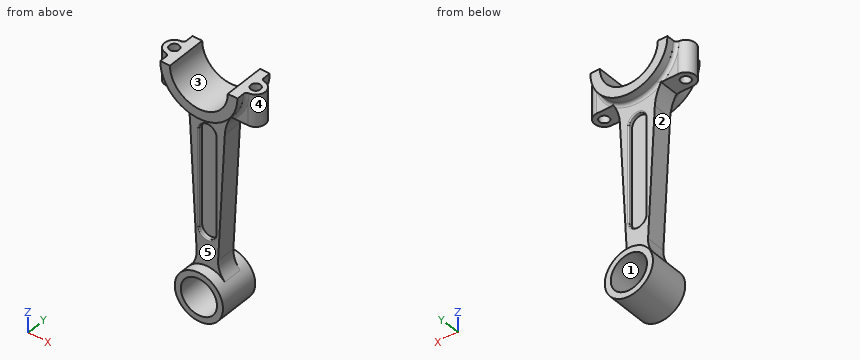
```python
from build123d import *

# Parameters (mm, degrees)
SKETCH1_R             = 22.5
SKETCH1_R_2           = 16.9
BOSS_EXTRUDE1_DEPTH   = 19
BOSS_EXTRUDE1_2_DEPTH = 19
BOSS_EXTRUDE2_DEPTH   = 9
BOSS_EXTRUDE3_DEPTH   = 5
FILLET2_R             = 1
BOSS_EXTRUDE4_DEPTH   = 9
FILLET3_R             = 3
SKETCH5_R             = 4.5
CUT_EXTRUDE1_DEPTH    = 38


with BuildPart() as part:
    # Sketch1 → Boss-Extrude1 (new, symmetric)
    with BuildSketch(Plane(origin=(0, 0, 0), x_dir=(1, 0, 0), z_dir=(0, 1, 0))):
        with Locations(Location((0, 201.2, 0), (0, 0, 270))):
            Circle(SKETCH1_R)
        with Locations(Location((0, 201.2, 0), (0, 0, 270))):
            Circle(SKETCH1_R_2, mode=Mode.SUBTRACT)
    extrude(amount=BOSS_EXTRUDE1_DEPTH, both=True)



with BuildPart() as body_2:
    # Sketch1 → Boss-Extrude1 2 (new, symmetric)
    with BuildSketch(Plane(origin=(0, 0, 0), x_dir=(1, 0, 0), z_dir=(0, 1, 0))):
        with BuildLine():
            Line((27, 0), (36, 0))
            ThreePointArc((36, 0), (0, 36), (-36, 0))
            Line((-36, 0), (-27, 0))
            ThreePointArc((-27, 0), (0, 27), (27, 0))
        make_face()
    extrude(amount=BOSS_EXTRUDE1_2_DEPTH, both=True)


with BuildPart() as part_1:
    add(part.part)

    add(body_2.part)  # Boss-Extrude2 merges body 2
    # Sketch1<3> → Boss-Extrude2 (add, symmetric)
    with BuildSketch(Plane(origin=(0, 0, 0), x_dir=(1, 0, 0), z_dir=(0, 1, 0))):
        with BuildLine():
            ThreePointArc((-16.279722223, 49.041287854), (-19.307974883, 35.735363352), (-26.63284908, 24.221712365))
            ThreePointArc((-26.63284908, 24.221712365), (0, 36), (26.63284908, 24.221712365))
            ThreePointArc((26.63284908, 24.221712365), (19.307974883, 35.735363352), (16.279722223, 49.041287854))
            Line((16.279722223, 49.041287854), (10, 168.865525948))
            ThreePointArc((10, 168.865525948), (11.381584619, 177.889356271), (16.234582266, 185.621542482))
            ThreePointArc((16.234582266, 185.621542482), (0, 178.7), (-16.234582266, 185.621542482))
            ThreePointArc((-16.234582266, 185.621542482), (-11.381584619, 177.889356271), (-10, 168.865525948))
            Line((-10, 168.865525948), (-16.279722223, 49.041287854))
        make_face()
        with BuildLine():
            ThreePointArc((8, 55.6), (0, 47.6), (-8, 55.6))
            Line((-8, 55.6), (-8, 145.6))
            ThreePointArc((-8, 145.6), (0, 153.6), (8, 145.6))
            Line((8, 145.6), (8, 55.6))
        make_face(mode=Mode.SUBTRACT)
    extrude(amount=BOSS_EXTRUDE2_DEPTH, both=True)

    # Sketch1<4> → Boss-Extrude3 (add, symmetric)
    with BuildSketch(Plane(origin=(0, 0, 0), x_dir=(1, 0, 0), z_dir=(0, 1, 0))):
        with BuildLine():
            Line((8, 55.6), (8, 145.6))
            ThreePointArc((8, 145.6), (0, 153.6), (-8, 145.6))
            Line((-8, 145.6), (-8, 55.6))
            ThreePointArc((-8, 55.6), (0, 47.6), (8, 55.6))
        make_face()
    extrude(amount=BOSS_EXTRUDE3_DEPTH, both=True)

    # Fillet2
    fillet2_edges = [part_1.edges().sort_by_distance(p)[0] for p in [
        (0, 9, -153.6),
        (8, 9, -100.6),
        (0, 9, -47.6),
        (-8, -9, -100.6),
        (-8, 9, -100.6),
        (0, -9, -153.6),
        (0, -9, -47.6),
        (8, -9, -100.6),
    ]]
    fillet(fillet2_edges, radius=FILLET2_R)

    # Sketch3 → Boss-Extrude4 (add, symmetric)
    with BuildSketch(Plane(origin=(0, 0, 0), x_dir=(1, 0, 0), z_dir=(0, 1, 0))):
        with BuildLine():
            Line((-19.899748742, 30), (-49, 30))
            Line((-49, 30), (-49, 0))
            Line((-49, 0), (-36, 0))
            ThreePointArc((-36, 0), (-31.720584442, 17.023645986), (-19.899748742, 30))
        make_face()
        with BuildLine():
            Line((49, 30), (49, 0))
            Line((49, 0), (36, 0))
            ThreePointArc((36, 0), (31.720584442, 17.023645986), (19.899748742, 30))
            Line((19.899748742, 30), (49, 30))
        make_face()
    extrude(amount=BOSS_EXTRUDE4_DEPTH, both=True)

    # Fillet3
    # the kernel refuses this fillet: 3 mm, written as the material it adds along each edge
    with BuildSketch(Plane(origin=(0, 9, 0), x_dir=(-1, 0, 0), z_dir=(0, 0, 1))) as fillet3_piece_1_section:
        with BuildLine():
            CenterArc((36 + FILLET3_R, -FILLET3_R), FILLET3_R, 90, 90)
            Line((36, -FILLET3_R), (36, 0))
            Line((36, 0), (36 + FILLET3_R, 0))
        make_face()
    fillet3_piece_1 = revolve(axis=Axis((0, 9, 0), (0, -1, 0)), revolution_arc=180, mode=Mode.PRIVATE)
    fillet3_piece_1 = split(fillet3_piece_1, bisect_by=Plane(origin=(-34.322989988, 9.698532199, -30), z_dir=(0, 0, 1)), keep=Keep.TOP, mode=Mode.PRIVATE)
    add(fillet3_piece_1)
    with BuildSketch(Plane(origin=(0, 9, 0), x_dir=(-1, 0, 0), z_dir=(0, 0, 1))) as fillet3_piece_2_section:
        with BuildLine():
            CenterArc((36 + FILLET3_R, -FILLET3_R), FILLET3_R, 90, 90)
            Line((36, -FILLET3_R), (36, 0))
            Line((36, 0), (36 + FILLET3_R, 0))
        make_face()
    fillet3_piece_2 = revolve(axis=Axis((0, 9, 0), (0, -1, 0)), revolution_arc=180, mode=Mode.PRIVATE)
    fillet3_piece_2 = fillet3_piece_2 - Plane(origin=(56.224903613, 10.5000003, -51.134726104), x_dir=(-0.7398013633284897, 0, 0.6728253434713263), z_dir=(0, 1, 0)) * Cylinder(40, 157, mode=Mode.PRIVATE)
    fillet3_piece_2 = fillet3_piece_2 - Plane(origin=(-56.224903613, 10.5000003, -51.134726104), x_dir=(0.9986295347545738, 0, 0.05233595624294564), z_dir=(0, 1, 0)) * Cylinder(40, 157, mode=Mode.PRIVATE)
    add(fillet3_piece_2)
    with BuildSketch(Plane(origin=(0, -9, 0), x_dir=(1, 0, 0), z_dir=(0, 0, 1))) as fillet3_piece_3_section:
        with BuildLine():
            CenterArc((36 + FILLET3_R, -FILLET3_R), FILLET3_R, 90, 90)
            Line((36, -FILLET3_R), (36, 0))
            Line((36, 0), (36 + FILLET3_R, 0))
        make_face()
    fillet3_piece_3 = revolve(axis=Axis((0, -9, 0), (0, 1, 0)), revolution_arc=180, mode=Mode.PRIVATE)
    fillet3_piece_3 = split(fillet3_piece_3, bisect_by=Plane(origin=(34.322988047, -9.698532268, -30), z_dir=(0, 0, 1)), keep=Keep.TOP, mode=Mode.PRIVATE)
    add(fillet3_piece_3)
    with BuildSketch(Plane(origin=(0, -9, 0), x_dir=(1, 0, 0), z_dir=(0, 0, 1))) as fillet3_piece_4_section:
        with BuildLine():
            CenterArc((36 + FILLET3_R, -FILLET3_R), FILLET3_R, 90, 90)
            Line((36, -FILLET3_R), (36, 0))
            Line((36, 0), (36 + FILLET3_R, 0))
        make_face()
    fillet3_piece_4 = revolve(axis=Axis((0, -9, 0), (0, 1, 0)), revolution_arc=180, mode=Mode.PRIVATE)
    fillet3_piece_4 = fillet3_piece_4 - Plane(origin=(56.224903613, -10.5000003, -51.134726104), x_dir=(-0.7398013633284897, 0, 0.6728253434713263), z_dir=(0, 1, 0)) * Cylinder(40, 157, mode=Mode.PRIVATE)
    fillet3_piece_4 = fillet3_piece_4 - Plane(origin=(-56.224903613, -10.5000003, -51.134726104), x_dir=(0.9986295347545738, 0, 0.05233595624294564), z_dir=(0, 1, 0)) * Cylinder(40, 157, mode=Mode.PRIVATE)
    add(fillet3_piece_4)

    # Sketch5 → Cut-Extrude1 (cut)
    with BuildSketch(Plane.XY):
        with BuildLine():
            Line((39, -9), (49, -9))
            Line((49, -9), (49, 9))
            Line((49, 9), (39, 9))
            Line((39, 9), (38, 9))
            ThreePointArc((38, 9), (47, 0), (38, -9))
            Line((38, -9), (39, -9))
        make_face()
        with BuildLine():
            ThreePointArc((-38, 9), (-47, 0), (-38, -9))
            Line((-38, -9), (-49, -9))
            Line((-49, -9), (-49, 9))
            Line((-49, 9), (-38, 9))
        make_face()
        with Locations((38, 0)):
            Circle(SKETCH5_R)
        with Locations((-38, 0)):
            Circle(SKETCH5_R)
    extrude(amount=-CUT_EXTRUDE1_DEPTH, mode=Mode.SUBTRACT)


solid = part_1.part
```
The model under review builds one solid part; all positions refer to its coordinate system, in mm. Face numbers are marked on the shaded views. A direction names the side the tool comes from. Round coordinates to 2 decimals unless told otherwise and drop trailing zeros. Write each loop counter-clockwise with the first axis right and the second up, starting at its lowest first coordinate (ties: lowest second). Pieces come first, ordered by that corner, then holes. Notation, with made-up numbers: (-8, 11) - (25, 11) arc R10 cw to (25, 23) - close; hole circle Ø11 at (-10.75, 8.25). An arc over 180 degrees is marked (long way). One line per question, with ' | ' between items.
Item 1: Add section C-C, the plane z = -102.5. Give the boundary of the cut face in (x, y), then the cut area to 3 significant figures.
Resolved:
outline: (-13.48, -9) - (-9, -9) arc R1 ccw to (-8, -8) - (-8, -5) - (8, -5) - (8, -8) arc R1 ccw to (9, -9) - (13.48, -9) - (13.48, 9) - (9, 9) arc R1 ccw to (8, 8) - (8, 5) - (-8, 5) - (-8, 8) arc R1 ccw to (-9, 9) - (-13.48, 9) - close | area: 356 mm2
Item 2: Add section D-D, the plane z = -172. Give the boundary of the cut face in (x, y).
Resolved:
outline: (-10.05, -9) - (10.05, -9) - (10.05, 9) - (-10.05, 9) - close
Item 3: To check wall thickness, follow probe 1 along X at (y, z) = (-10, -201.2); probe 2 along Z at (x, y) = (-12, -10); probe 3 along Y at (x, z) = (32.5, -21.5). State the ranges of each line that lie inside material, in increasing order.
Resolved:
probe 1: x = -22.5 to -16.9, 16.9 to 22.5 | probe 2: z = -220.23 to -213.1, -189.3 to -182.17, -34.75 to -24.19 | probe 3: y = -9 to 9
Item 4: Add section B-B, the plane z = -206. Give the boundary of the cut face in (x, y), then the cut area to 3 significant figures.
Resolved:
outline: (-21.98, -19) - (-16.2, -19) - (-16.2, 19) - (-21.98, 19) - close; (16.2, -19) - (21.98, -19) - (21.98, 19) - (16.2, 19) - close | area: 439 mm2
Item 5: For P1, Ø14.5, axis at x = 38, y = 0, coming from the -Z side; P2, Ø1.5, axis at y = -6, z = -82.5, coming from the +X side; P3, Ø8, axis at x = -2.5, y = 2, coming from the +Z side, all flat-tipped, find the tip position at first contact; note any pin that passes through.
Resolved:
P1: stops at z = -30 | P2: stops at x = 14.57 | P3: stops at z = -26.21
Item 6: For the marked faces 1 and 2, list the 3-axis set-ups (+Z, -Z, +X, -X, +Y, -Y) from which the entire face can be reached by the end or side of a thin tool; tool diameter is ignored.
Resolved:
face 1: +Y, -Y | face 2: -X, +Y, -Y
Item 7: The part is to be moulded in two halves that separate along X. For the marked faces 3, 4 and 5, say which applies: pulls with the +X half, pulls with the -X half, needs draft (parallel to the pull), parting line crosses it, or undercut.
Resolved:
face 3: undercut | face 4: pulls with the +X half | face 5: needs draft
Item 8: Add section A-A, the plane y = 16. Give the boundary of the cut face in (x, z), then the cut area to 3 significant figures.
Resolved:
outline: (-36, 0) arc R36 ccw to (36, 0) - (27, 0) arc R27 cw to (-27, 0) - close; circle Ø45 at (0, -201.2); hole circle Ø33.8 at (0, -201.2) | area: 1,580 mm2
